Read the model definition and answer for the solid it produces. Units are mm, in the model's axes. A direction names the side the tool comes from. Coordinates: 2 decimals unless noted, no trailing zeros. Write each loop counter-clockwise with the first axis right and the second up, starting at its lowest first coordinate (ties: lowest second). Pieces come first, ordered by that corner, then holes.
1) Each of these flat-tipped pins is pushed along its axis until it touches: pin 1 Ø6 at (x, z) = (-38.5, -4) entering from -Y; pin 2 Ø10 at (x, z) = (-1, -1) entering from -Y; pin 3 Ø4 at (x, z) = (17.5, 4) entering from +Y; pin 4 Ø6 at (y, z) = (-1.5, 2) entering from -X (3 decimals). Where does it stop, or does it pass through?
2) The part is cut by section C-C (x = -38). Determine the outline of the cut face in (y, z), then the cut area to 3 significant figures.
3) Find the intervals of material crossed by line 1 (Z direction, x = 8, y = -0.5); line 2 (Y direction, x = -25, z = 3.5); line 3 (Y direction, x = -40, z = -4), in increasing order.
4) The part is cut by section D-D (x = 23). Determine the outline of the cut face in (y, z), then the cut area to 3 significant figures.
5) Which of the six approach directions +Z, -Z, +X, -X, +Y, -Y give full straight-line access (tool end or side, diameter ignored) to faces 1 (the face through (-47.142, 2.285, 3.584)), 2 (the face through (-11.737, 4.57, 7.167)), 3 (the face through (-32.54, -2.01, -9.03))?
from build123d import *


with BuildPart() as part:
    # Sketch1 → Revolve1 (revolve)
    with BuildSketch(Plane.XY):
        with BuildLine():
            Line((-49.375, 0), (49.375, 0))
            Line((49.375, 0), (49.375, 3))
            Line((49.375, 3), (17.375, 3))
            Line((17.375, 3), (17.375, 7.5))
            Line((17.375, 7.5), (2.375, 7.5))
            Line((2.375, 7.5), (-3.625, 8.5))
            Line((-3.625, 8.5), (-19.625, 8.5))
            Line((-19.625, 8.5), (-20.375, 9.25))
            Line((-20.375, 9.25), (-44.375, 9.25))
            Line((-44.375, 9.25), (-45.875, 4.25))
            Line((-45.875, 4.25), (-48.375, 4.25))
            ThreePointArc((-48.375, 4.25), (-49.121632386, 2.18303115), (-49.375, 0))
        make_face()
    revolve(axis=Axis((0, 0, 0), (1, 0, 0)))


solid = part.part
Reported:
1. pin 1: stops at y = -9.2
1. pin 2: stops at y = -8.5
1. pin 3: stops at y = 7.23
1. pin 4: stops at x = -49.375
2. outline: circle Ø18.5 at (0, 0)
2. area: 269 mm2
3. line 1: z = -7.48 to 7.48
3. line 2: y = -8.56 to 8.56
3. line 3: y = -8.34 to 8.34
4. outline: circle Ø6 at (0, 0)
4. area: 28.3 mm2
5. face 1: -X
5. face 2: +X
5. face 3: +X, -X
